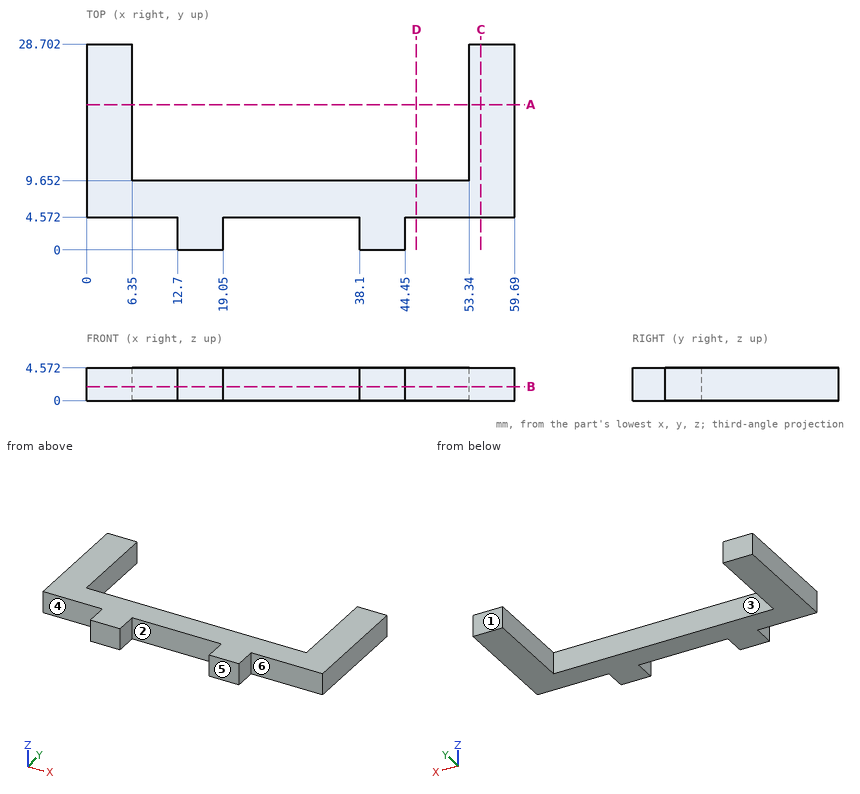
Can you work these out from the drawing? Everything is in mm from the part's minimum corner. A direction names the side the tool comes from. Give positions to 0.01 mm unless a question says otherwise; leave off trailing zeros. Loops run counter-clockwise (first coordinate to the right, second up) from the corner with the lowest first, then second, coordinate; pieces in that order, holes last. Notation, with made-up numbers: (-26, 14) -> (-11, 14) arc R21 ccw to (-11, 31) -> close; hole circle Ø5 at (-38.5, 64.25). An arc over 180 degrees is marked (long way). Write item = value, one per line.
1) Suppose I cut it at D-D on x = 46. Write out the boundary of the cut face in (y, z).
Check result:
outline = (4.57, 0) -> (9.65, 0) -> (9.65, 4.57) -> (4.57, 4.57) -> close
2) I need wall thicknesses on L1, parallel to X at y = 16, z = 0.4; L2, parallel to X at y = 4, z = 2.5; L3, parallel to Y at x = 3.5, z = 1.15. Which ranges of each line are inside material? Lowest first, please. Write a range as from..to.
Check result:
L1 = 0..6.35, 53.34..59.69
L2 = 12.7..19.05, 38.1..44.45
L3 = 4.57..28.7
3) For the marked faces 3, 4, 5 and 6, which set-ups out of +Z, -Z, +X, -X, +Y, -Y let a thin tool reach every point of the face, with its end or its side?
Check result:
face_3 = +Z, -Z, +Y
face_4 = +Z, -Z, -X, -Y
face_5 = +Z, -Z, +X, -X, -Y
face_6 = +Z, -Z, +X, -Y
4) Suppose I cut it at A-A on y = 20.25. Write out the boundary of the cut face in (x, z), then the cut area to 3 significant figures.
Check result:
outline = (0, 0) -> (6.35, 0) -> (6.35, 4.57) -> (0, 4.57) -> close; (53.34, 0) -> (59.69, 0) -> (59.69, 4.57) -> (53.34, 4.57) -> close
area = 58.1 mm2
5) Suppose I cut it at B-B on z = 1.95. Write out the boundary of the cut face in (x, y).
Check result:
outline = (0, 4.57) -> (12.7, 4.57) -> (12.7, 0) -> (19.05, 0) -> (19.05, 4.57) -> (38.1, 4.57) -> (38.1, 0) -> (44.45, 0) -> (44.45, 4.57) -> (59.69, 4.57) -> (59.69, 28.7) -> (53.34, 28.7) -> (53.34, 9.65) -> (6.35, 9.65) -> (6.35, 28.7) -> (0, 28.7) -> close
6) Will these pins go through, and if not, where does the flat tip stop? pin 1 (1.4 mm diameter, centred on y = 2.5, z = 2.5, fed in from -X); pin 2 (1.5 mm diameter, centred on x = 50, z = 1.5, fed in from +Y); pin 3 (2.5 mm diameter, centred on x = 53, z = 3.5, fed in from -Y).
Check result:
pin_1 = 12.7
pin_2 = 9.65
pin_3 = 4.57
7) Thinking about a two-plate mould opening in X: for the marked faces 1 and 2, which applies, released by +X, released by -X, zero draft, split by the parting line, or undercut?
Check result:
face_1 = zero draft
face_2 = undercut
8) Suppose I cut it at C-C on x = 55. Write out the boundary of the cut face in (y, z).
Check result:
outline = (4.57, 0) -> (28.7, 0) -> (28.7, 4.57) -> (4.57, 4.57) -> close
